Could you check a few things on this model? Use its own coordinates, in mm. A direction names the side the tool comes from. Coordinates: 2 decimals unless noted, no trailing zeros. Write each loop counter-clockwise with the first axis right and the second up, starting at its lowest first coordinate (ties: lowest second). Pieces come first, ordered by that corner, then holes. Notation, with made-up numbers: M -2.75,9.25 L 53.25,9.25 A24 ccw 53.25,36.25 Z; hole C -37,65 d6. An arc over 180 degrees is marked long. Answer as CSV lines item,"result". Start each with the question number.
Item 1: I'm going to push flat-ended pins straight in: P1, Ø2.5, axis at y = 39.61, z = -61.35, coming from the +X side; P2, Ø1, axis at x = 82.5, y = 46.5, coming from the -Z side; P3, Ø5, axis at y = 142, z = -84.6, coming from the +X side. Where does each tip first touch, or does it pass through?
Item 2: On a 3-axis mill with a long thin cutter (end or side, diameter ignored), from which of +Z, -Z, +X, -X, +Y, -Y can I reach the whole of each face in a straight line? I mean faces 4 (the cylindrical face through (3.13, 148.02, -58.87)), 5 (the flat face through (39, 150, -6)), 6 (the flat face through (55, 74, -6.35)). Say none if no direction works.
Item 3: Suppose I cut it at C-C, the plane y = 32. Write out the boundary of the cut face in (x, z), and give its area (3 significant figures).
Item 4: If I drill on line 1 along Y through (x, z) = (2, -49.6); line 2 along Y through (x, z) = (2, -57); line 3 along Y through (x, z) = (91, -4), over which ranges is the centre line in solid material (lowest first)? Write a range as [from, to].
Item 5: Suppose I cut it at B-B, the plane x = 91.6. Write out the boundary of the cut face in (y, z).
Item 6: Suppose I cut it at A-A, the plane z = -84.6. Write out the boundary of the cut face in (x, y), and give its area (3 significant figures).
Item 7: We'd pull the mould along X, two halves only. Please class faces 1 (the flat face through (101.6, 74, -3)), 2 (the cylindrical face through (3.131, 140.226, -13.677)), 3 (the cylindrical face through (10, 77, -3)): +X half, -X half, draft (parallel to the pull), parting line (faces both ways), or undercut.
Item 8: Suppose I cut it at D-D, the plane x = 78. Write out the boundary of the cut face in (y, z), and give its area (4 significant figures).
```python
from build123d import *

# Parameters (mm, degrees)
SALIENTE_EXTRUIR1_DEPTH = 150
CROQUIS2_R              = 2
CROQUIS2_R_2            = 11
CROQUIS2_R_3            = 1.5
CROQUIS2_R_4            = 6
CORTAR_EXTRUIR1_DEPTH   = 208.714034191
REDONDEO1_R             = 10
CROQUIS3_R              = 12.5
CORTAR_EXTRUIR2_DEPTH   = 1.5
CROQUIS4_R              = 2
CROQUIS4_R_2            = 1.5
CORTAR_EXTRUIR3_DEPTH   = 208.714034191
CROQUIS6_R              = 2
CORTAR_EXTRUIR4_DEPTH   = 208.714034191


with BuildPart() as part:
    # Croquis1 → Saliente-Extruir1 (new body)
    with BuildSketch(Plane(origin=(0, 0, 0), x_dir=(1, 0, 0), z_dir=(0, 1, 0))):
        Polygon((0, 101.6), (0, 0), (101.6, 0), (101.6, 6.35), (6.35, 6.35), (6.35, 101.6), align=None)
    extrude(amount=SALIENTE_EXTRUIR1_DEPTH)

    # Croquis2 → Cortar-Extruir1 (cut, through all)
    with BuildSketch(Plane.ZY):
        with Locations((-84.6, 142)):
            Circle(CROQUIS2_R)
        with Locations((-14.6, 142)):
            Circle(CROQUIS2_R)
        with Locations((-49.6, 59.96)):
            Circle(CROQUIS2_R_2)
        with Locations((-49.6, 7.71)):
            Circle(CROQUIS2_R_3)
        with Locations((-49.6, 144.86)):
            Circle(CROQUIS2_R_4)
        with Locations((-49.6, 106.86)):
            Circle(CROQUIS2_R_4)
    extrude(amount=-CORTAR_EXTRUIR1_DEPTH, mode=Mode.SUBTRACT)

    # Redondeo1
    redondeo1_edges = [part.edges().sort_by_distance(p)[0] for p in [
        (3.175, 150, -52.695222125),
        (3.175, 150, -46.504777875),
    ]]
    fillet(redondeo1_edges, radius=REDONDEO1_R)

    # Croquis3 → Cortar-Extruir2 (cut)
    with BuildSketch(Plane.ZY):
        with Locations((-49.6, 59.96)):
            Circle(CROQUIS3_R)
    extrude(amount=-CORTAR_EXTRUIR2_DEPTH, mode=Mode.SUBTRACT)

    # Croquis4 → Cortar-Extruir3 (cut, through all)
    with BuildSketch(Plane.ZY):
        with Locations((-49.6, 78.61)):
            Circle(CROQUIS4_R)
        with Locations((-49.6, 41.31)):
            Circle(CROQUIS4_R)
        with Locations((-34.6, 59.96)):
            Circle(CROQUIS4_R_2)
        with Locations((-57.1, 46.969618943)):
            Circle(CROQUIS4_R_2)
        with Locations((-57.1, 72.950381057)):
            Circle(CROQUIS4_R_2)
        with Locations((-26.1, 59.96)):
            Circle(CROQUIS4_R_2)
        with Locations((-61.35, 39.608403011)):
            Circle(CROQUIS4_R_2)
        with Locations((-61.35, 80.311596989)):
            Circle(CROQUIS4_R_2)
    extrude(amount=-CORTAR_EXTRUIR3_DEPTH, mode=Mode.SUBTRACT)

    # Croquis6 → Cortar-Extruir4 (cut, through all)
    with BuildSketch(Plane.XY):
        with Locations((91.6, 140)):
            Circle(CROQUIS6_R)
        with Locations((91.6, 75)):
            Circle(CROQUIS6_R)
        with Locations((91.6, 10)):
            Circle(CROQUIS6_R)
        with Locations((10, 10)):
            Circle(CROQUIS6_R)
        with Locations((10, 75)):
            Circle(CROQUIS6_R)
        with Locations((10, 140)):
            Circle(CROQUIS6_R)
    extrude(amount=-CORTAR_EXTRUIR4_DEPTH, mode=Mode.SUBTRACT)


solid = part.part
```
Ans:
1,P1,"passes through"
1,P2,"stops at z = -6.35"
1,P3,"stops at x = 6.35"
2,face 4,"+X, -X, +Y"
2,face 5,"+Z, -Z, +X, -X, +Y"
2,face 6,"-Z, +X, +Y, -Y"
3,outline,"M 0,-101.6 L 6.35,-101.6 L 6.35,-6.35 L 101.6,-6.35 L 101.6,0 L 0,0 Z"
3,area,"1,250 mm^2"
4,line 1,"y = [0, 6.21], [9.21, 39.31], [43.31, 48.96], [70.96, 76.61], [80.61, 100.86], [112.86, 138.86]"
4,line 2,"y = [0, 45.47], [48.47, 51.82], [68.1, 71.45], [74.45, 146.2]"
4,line 3,"y = [0, 8.09], [11.91, 73.09], [76.91, 138.09], [141.91, 150]"
5,outline,"M 0,-6.35 L 8,-6.35 L 8,0 L 0,0 Z; M 12,-6.35 L 73,-6.35 L 73,0 L 12,0 Z; M 77,-6.35 L 138,-6.35 L 138,0 L 77,0 Z; M 142,-6.35 L 150,-6.35 L 150,0 L 142,0 Z"
6,outline,"M 0,0 L 6.35,0 L 6.35,140 L 0,140 Z; M 0,144 L 6.35,144 L 6.35,150 L 0,150 Z"
6,area,"927 mm^2"
7,face 1,"+X half"
7,face 2,"draft"
7,face 3,"undercut"
8,outline,"M 0,-6.35 L 150,-6.35 L 150,0 L 0,0 Z"
8,area,"952.5 mm^2"
